Autodesk Inventor part; units mm, degrees
ref_plane "YZ Plane" through (0, 0, 0) normal (1, 0, 0) x (0, 1, 0)
ref_plane "XZ Plane" through (0, 0, 0) normal (0, 1, 0) x (-1, 0, 0)
ref_plane "XY Plane" through (0, 0, 0) normal (0, 0, 1) x (1, 0, 0)
sketch "草图1" plane through (0, 0, 0) normal (0, 1, 0) x (-1, 0, 0)
  line L0 (0, 0) -> (-15, 0) construction
  line L1 (0, 2) -> (-15, 2)
  line L2 (-15, -2) -> (0, -2)
  arc A0 (0, -2) -> (0, 2) centre (0, 0) ccw
  arc A1 (-15, 2) -> (-15, -2) centre (-15, 0) ccw
  line L3 (-15, 0) -> (-19.5, -7.7942) construction
  line L4 (-13.2679, -1) -> (-17.7679, -8.7942)
  line L5 (-21.2321, -6.7942) -> (-16.7321, 1)
  arc A2 (-13.2679, -1) -> (-16.7321, 1) centre (-15, 0) ccw
  arc A3 (-21.2321, -6.7942) -> (-17.7679, -8.7942) centre (-19.5, -7.7942) ccw
  line L6 (-15, 0) -> (-6, 0) construction
  circle A4 centre (0, 0) radius 1
  point P0 (-7.5, 0)
  point P1 (-17.25, -3.8971)
  point P2 (-16.7321, 1)
  point P3 (-13.8453, -2)
  dimension "d0" = 15
  dimension "d1" = 2
  dimension "d2" = 9
  dimension "d3" = 120
  dimension "d4" = 2
extrude "拉伸1" add sketch "草图1" along normal blind 3
properties part number "夹爪01"
Build history of the part. All positions in model axes, mm. A direction names the side the tool comes from. Round coordinates to 2 decimals unless told otherwise and drop trailing zeros. Loops run counter-clockwise (first coordinate to the right, second up) from the corner with the lowest first, then second, coordinate; pieces in that order, holes last. Notation, with made-up numbers: M 43.5,-3 L 63.5,-3 A19 ccw 63.5,19 Z; hole C 58.25,-30 d10. An arc over 180 degrees is marked long. Answer as CSV lines item,"result".
1. Two-plate mould, pull along X, no slides. Class faces 3 (the cylindrical face through (20.46, 1.48, -9.55)), 4 (the flat face through (7, 1, 2)), 5 (the cylindrical face through (0, 1, 1)): released by +X, released by -X, zero draft, split by the parting line, or undercut.
Resolved:
face 3,"split by the parting line"
face 4,"zero draft"
face 5,"undercut"
2. Cut at A-A on y = 1.8. Write the cut outline in (x, z), then the cut area to 3 significant figures.
Resolved:
outline,"M 0,-2 L 13.85,-2 L 17.77,-8.79 A2 ccw 21.23,-6.79 L 16.73,1 A2 ccw 15,2 L 0,2 A2 ccw Z; hole C 0,0 d2"
area,"105 mm²"
3. Wall check: probe 1 along Z at (x, y) = (0, 1.45); probe 2 along Z at (x, y) = (12, 2.25); probe 3 along X at (y, z) = (2.75, 0.25). Give the ranges that are in metal, low to high. Write a range as [from, to].
Resolved:
probe 1,"z = [-2, -1], [1, 2]"
probe 2,"z = [-2, 2]"
probe 3,"x = [-1.98, -0.97], [0.97, 17.17]"
4. Cut at C-C on x = 1.25. Write the cut outline in (y, z), then the cut area to 3 significant figures.
Resolved:
outline,"M 0,-2 L 3,-2 L 3,2 L 0,2 Z"
area,"12.0 mm²"
5. Flat gauge pins, fed straight in: P1, Ø3, axis at x = 7, z = 0.5, coming from the -Y side; P2, Ø1.5, axis at x = 3.5, y = 1, coming from the -Z side. Where does each tip first touch, or does it go through?
Resolved:
P1,"stops at y = 0"
P2,"stops at z = -2"
6. Cut at B-B on z = 0. Write the cut outline in (x, y).
Resolved:
outline,"M -2,0 L -1,0 L -1,3 L -2,3 Z; M 1,0 L 17.31,0 L 17.31,3 L 1,3 Z"
7. Cut at D-D on z = -8. Write the cut outline in (x, y).
Resolved:
outline,"M 17.31,0 L 21.49,0 L 21.49,3 L 17.31,3 Z"
8. 3-axis set-ups, long thin cutter, end or side, ignore diameter. For faces 1 (the flat face through (13, 3, -1)), 2 (the flat face through (7, 1, -2)): which of +Z, -Z, +X, -X, +Y, -Y reach the whole face in a straight line?
Resolved:
face 1,"+Z, -Z, +X, -X, +Y"
face 2,"-Z, -X, +Y, -Y"
